Input: dimensioned drawing with shaded views. Units: mm. Origin: part minimum x, y, z. A direction names the side the tool comes from. Give positions to 0.01 mm unless a question says otherwise; leave off trailing zeros. Loops run counter-clockwise (first coordinate to the right, second up) from the corner with the lowest first, then second, coordinate; pieces in that order, holes last. Notation, with made-up numbers: (82.25, 80.5) -> (96.25, 80.5) arc R22 ccw to (96.25, 112.5) -> close; hole circle Ø7 at (15, -30). An arc over 180 degrees is marked (long way). One line per question, with ' | ' between items. Start each with the question number.
Item 1: Section B-B on x = 9.5. Return loops of the section in (y, z).
Item 2: Set-up query: the marked faces 4, 5 and 6. Return all of +Z, -Z, +X, -X, +Y, -Y with unobstructed straight access to the full face (end or side cutting, diameter ignored); none if empty.
Item 3: Material intervals for line 1 along Z through (x, y) = (16, 68.5); line 2 along Y through (x, z) = (1.25, 38.5); line 3 along X through (y, z) = (9, 32), sorted ascending. Write a range as [from, to].
Item 4: Mould query, pull axis Z, two halves, no side actions, for the marked faces 1, 2 and 3. Classes: released by +Z, released by -Z, zero draft, split by the parting line, or undercut.
Item 5: Section D-D on y = 7.5. Return loops of the section in (x, z).
Item 6: Section C-C on y = 78.5. Return loops of the section in (x, z).
Item 7: Pin query (flat end, axial travel): P1, Ø4, axis at x = 8.5, y = 83, coming from the -Z side; P2, Ø1, axis at y = 11, z = 9, coming from the +X side. Return the tip coordinate at first contact, or that it passes through.
Item 8: Section A-A on z = 24. Return loops of the section in (x, y).
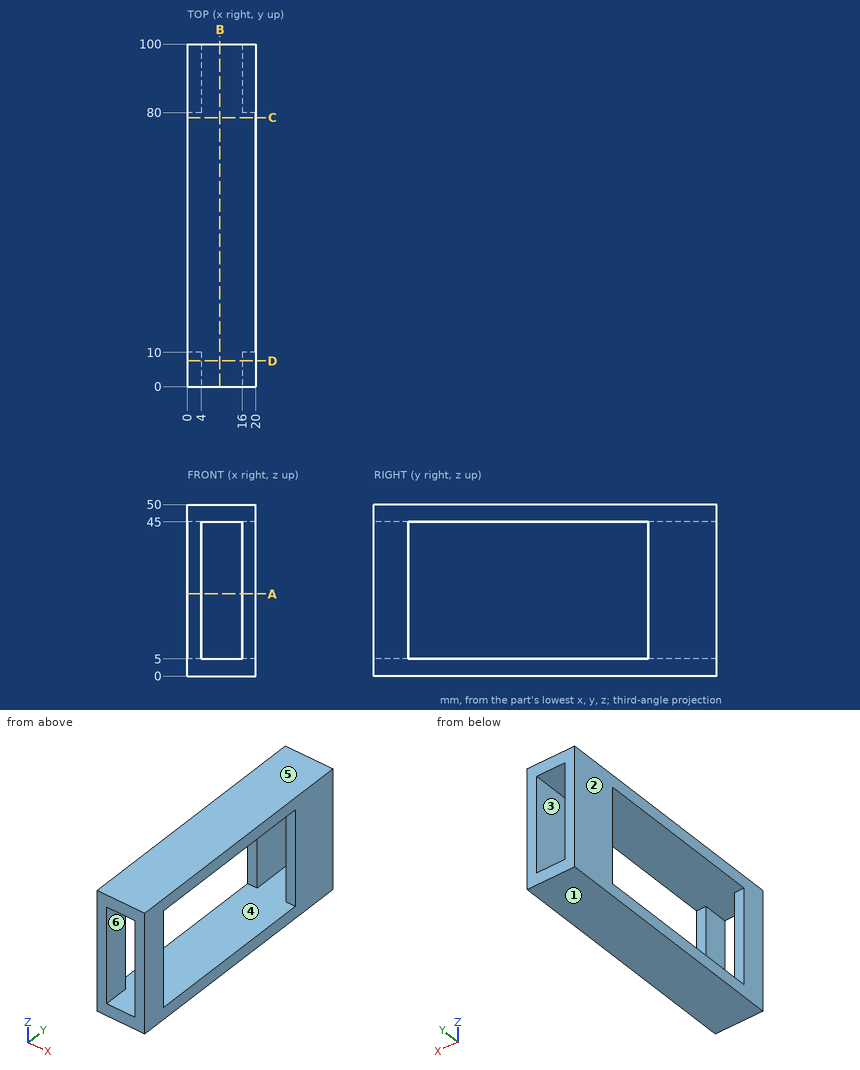
Result sheet:
1) outline: (0, 0) -> (100, 0) -> (100, 5) -> (0, 5) -> close; (0, 45) -> (100, 45) -> (100, 50) -> (0, 50) -> close
2) face 4: none | face 5: +Z, +X, -X, +Y, -Y | face 6: +Y, -Y
3) line 1: z = [0, 5], [45, 50] | line 2: y = [0, 10], [80, 100] | line 3: x = [0, 4], [16, 20]
4) face 1: released by -Z | face 2: zero draft | face 3: undercut
5) outline: (0, 0) -> (20, 0) -> (20, 50) -> (0, 50) -> close; hole (4, 5) -> (16, 5) -> (16, 45) -> (4, 45) -> close
6) outline: (0, 0) -> (20, 0) -> (20, 5) -> (0, 5) -> close; (0, 45) -> (20, 45) -> (20, 50) -> (0, 50) -> close
7) P1: stops at z = 0 | P2: passes through
8) outline: (0, 0) -> (4, 0) -> (4, 10) -> (0, 10) -> close; (0, 80) -> (4, 80) -> (4, 100) -> (0, 100) -> close; (16, 0) -> (20, 0) -> (20, 10) -> (16, 10) -> close; (16, 80) -> (20, 80) -> (20, 100) -> (16, 100) -> close
